Input: part model. Units: mm. Frame: model coordinates. Coordinates: 2 decimals unless noted, no trailing zeros. Write each loop counter-clockwise with the first axis right and the second up, starting at its lowest first coordinate (ties: lowest second). Pieces come first, ordered by that corner, then holes.
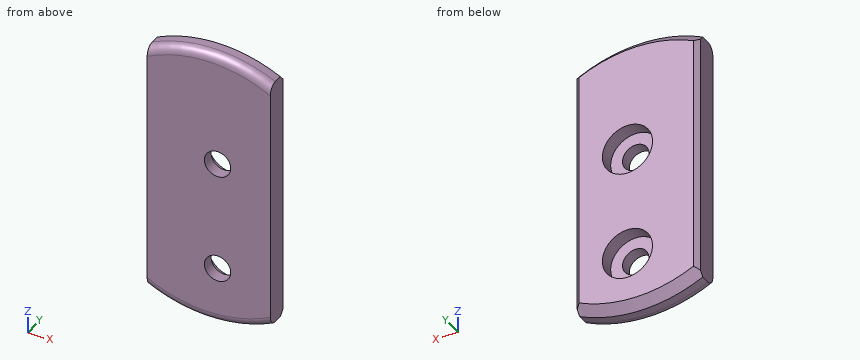
from build123d import *

# Parameters (mm, degrees)
SKETCH2_R           = 16
BOSS_EXTRUDE1_DEPTH = 3
SKETCH1_W           = 9
SKETCH1_H           = 32
CUT_EXTRUDE1_DEPTH  = 4
SKETCH3_R           = 1.5
CUT_EXTRUDE2_DEPTH  = 4
SKETCH4_R           = 2.85
CUT_EXTRUDE3_DEPTH  = 1.65
CHAMFER1_SIZE       = 0.5
FILLET1_R           = 1
CHAMFER2_SIZE       = 1


with BuildPart() as part:
    # Sketch2 → Boss-Extrude1 (new body)
    with BuildSketch(Plane(origin=(0, 0, 0), x_dir=(1, 0, 0), z_dir=(0, 1, 0))):
        Circle(SKETCH2_R)
    extrude(amount=BOSS_EXTRUDE1_DEPTH)

    # Sketch1 → Cut-Extrude1 (cut, through all)
    with BuildSketch(Plane(origin=(0, 0, 0), x_dir=(1, 0, 0), z_dir=(0, 1, 0))):
        with Locations((-11.5, 0)):
            Rectangle(SKETCH1_W, SKETCH1_H)
        with Locations((11.5, 0)):
            Rectangle(SKETCH1_W, SKETCH1_H)
    extrude(amount=CUT_EXTRUDE1_DEPTH, mode=Mode.SUBTRACT)

    # Sketch3 → Cut-Extrude2 (cut, through all)
    with BuildSketch(Plane(origin=(0, 3, 0), x_dir=(1, 0, 0), z_dir=(0, 1, 0))):
        with Locations((1, 9.4472)):
            Circle(SKETCH3_R)
        with Locations((1, -3.0528)):
            Circle(SKETCH3_R)
    extrude(amount=-CUT_EXTRUDE2_DEPTH, mode=Mode.SUBTRACT)

    # Sketch4 → Cut-Extrude3 (cut)
    with BuildSketch(Plane(origin=(0, 3, 0), x_dir=(1, 0, 0), z_dir=(0, 1, 0))):
        with Locations((1, 9.4472)):
            Circle(SKETCH4_R)
        with Locations((1, -3.0528)):
            Circle(SKETCH4_R)
    extrude(amount=-CUT_EXTRUDE3_DEPTH, mode=Mode.SUBTRACT)

    # Chamfer1
    chamfer1_edges = [part.edges().sort_by_distance(p)[0] for p in [
        (-7, 3, 0),
        (7, 3, 0),
    ]]
    chamfer(chamfer1_edges, length=CHAMFER1_SIZE)

    # Fillet1
    fillet1_edges = [part.edges().sort_by_distance(p)[0] for p in [
        (0, 0, -16),
        (0, 0, 16),
    ]]
    fillet(fillet1_edges, radius=FILLET1_R)

    # Chamfer2
    chamfer2_edges = [part.edges().sort_by_distance(p)[0] for p in [
        (0, 3, -16),
        (0, 3, 16),
    ]]
    chamfer(chamfer2_edges, length=CHAMFER2_SIZE)


solid = part.part
Item 1: Section query B-B, the plane y = 0.55. Return loops of the section in (x, z).
Item 2: Section query A-A, the plane z = -8.5. Return loops of the section in (x, y), then the cut area to 3 significant figures.
Item 3: Pin query (flat end, axial travel): pin 1 Ø4 at (x, z) = (1, 3.05) entering from -Y; pin 2 Ø3.5 at (x, z) = (1, 3.05) entering from +Y. Return the tip coordinate at first contact, or that it passes through.
Item 4: Material intervals for line 1 (Z direction, x = 1, y = 2.4); line 2 (Z direction, x = -0.25, y = 0.5); line 3 (Y direction, x = 2.5, z = 5), sorted ascending.
Item 5: Section query C-C, the plane x = 1. State how many separate pieces and enclosed holes the cut face has, then the cut area to 3 significant figures.
The answers:
1. outline: (-7, -14.27) arc R15.89 ccw to (7, -14.27) - (7, 14.27) arc R15.89 ccw to (-7, 14.27) - close; hole circle Ø3 at (1, -9.45); hole circle Ø3 at (1, 3.05)
2. outline: (-7, 0) - (-0.16, 0) - (-0.16, 1.35) - (-1.69, 1.35) - (-1.69, 3) - (-6.5, 3) - (-7, 2.5) - close; (2.16, 0) - (7, 0) - (7, 2.5) - (6.5, 3) - (3.69, 3) - (3.69, 1.35) - (2.16, 1.35) - close
2. area: 29.7 mm2
3. pin 1: stops at y = 0
3. pin 2: stops at y = 1.35
4. line 1: z = -15.57 to -12.3, -6.6 to 0.2, 5.9 to 15.57
4. line 2: z = -15.86 to -10.28, -8.62 to 2.22, 3.88 to 15.86
4. line 3: y = 0 to 1.35
5. separate pieces: 3
5. enclosed holes: 0
5. area: 67.5 mm2
